Input: part model. Units: mm. Frame: model coordinates. A direction names the side the tool comes from. Coordinates: 2 decimals unless noted, no trailing zeros. Order: outer loops, then holes, each group sorted by start corner. A loop starts at its lowest first (then second) coordinate and runs counter-clockwise, first axis right, second up. Notation, with made-up numbers: M 48,-20 L 53,-20 A12 cw 53,-5 Z; hole C -8,35.5 d2. An arc over 180 degrees is marked long. One line per item, written item: value.
```python
from build123d import *

# Parameters (mm, degrees)
F0_W     = 18.0536359549
F0_H     = 24.487555027
F1_DEPTH = 48.0590760708
F2_R     = 4.7851705696
F3_DEPTH = 59.6192404628
F4_SIZE  = 5.08
F5_T     = -2.54


with BuildPart() as f1:
    # F0 (on Top) → F1 (new body)
    with BuildSketch(Plane.XY):
        with Locations((-3.9722770452, 28.8042277098)):
            Rectangle(F0_W, F0_H)
    extrude(amount=F1_DEPTH)

    # F2 (on face) → F3 (cut)
    with BuildSketch(Plane.YZ.offset(5.0545409322)):
        with Locations((27.5146439672, 27.5505185127)):
            Circle(F2_R)
    extrude(amount=-F3_DEPTH, mode=Mode.SUBTRACT)

    # F4
    f4_edges = [f1.edges().sort_by_distance(p)[0] for p in [
        (5.054541, 28.804228, 48.059076),
    ]]
    chamfer(f4_edges, length=F4_SIZE)

    # F5
    f5_openings = [f1.faces().sort_by_distance(p)[0] for p in [
        (-12.999095, 40.508625, 24.029538),
    ]]
    offset(amount=F5_T, openings=f5_openings)


solid = f1.part
```
(1) Draft query along Y for faces 1 (the flat face through (2.515, 29, 18)), 2 (the flat face through (-4, 41.048, 24)), 3 (the flat face through (-12.999, 29, 32.3)), 4 (the flat face through (-4, 16.56, 24)). Return one class per face: released by +Y, released by -Y, zero draft, split by the parting line, or undercut.
Data:
face 1: undercut
face 2: released by +Y
face 3: zero draft
face 4: released by -Y
(2) Ray query, line 1 (Y direction, x = 0.5, z = 39); line 2 (Z direction, x = -8.25, y = 37.75); line 3 (Z direction, x = 2.25, y = 31.25). Return the intervals inside material, ascending. Write a range as from..to.
Data:
line 1: y = 16.56..19.1, 38.51..41.05
line 2: z = 0..2.54, 45.52..48.06
line 3: z = 0..2.54, 21.25..24.56, 30.54..33.85, 42.19..45.78
(3) First-contact query: pin 1 (4 mm diameter, centred on y = 35, z = 20.5, fed in from -X). Flat tip, straight axial feed; report the tip coordinate or a pass-through.
Data:
pin 1: stops at x = 2.51
(4) Cut plane A-A on x = 0.75. Output: boundary loops of the cut face in (y, z).
Data:
outline: M 16.56,0 L 41.05,0 L 41.05,47.28 L 16.56,47.28 Z; C 27.51,27.55 d14.65; hole M 19.1,2.54 L 38.51,2.54 L 38.51,43.69 L 19.1,43.69 Z; hole C 27.51,27.55 d9.57
(5) Access query for faces 5 (the flat face through (-5, 38.508, 24)), 6 (the flat face through (2.55, 28.633, 45.484)). Directions: +Z, -Z, +X, -X, +Y, -Y. A direction counts if a zero-diameter tool reaches every point of the face in a straight line with its end or side. Return the directions, or none.
Data:
face 5: -X
face 6: +Z, +X, +Y, -Y
(6) Cut plane C-C on z = 15.5. Output: boundary loops of the cut face in (x, y).
Data:
outline: M -13,16.56 L 5.05,16.56 L 5.05,41.05 L -13,41.05 L -13,38.51 L 2.51,38.51 L 2.51,19.1 L -13,19.1 Z
(7) Cut plane D-D on x = -10.25. Output: boundary loops of the cut face in (y, z), plus the area to 3 significant figures.
Data:
outline: M 16.56,0 L 41.05,0 L 41.05,48.06 L 16.56,48.06 Z; C 27.51,27.55 d14.65; hole M 19.1,2.54 L 38.51,2.54 L 38.51,45.52 L 19.1,45.52 Z; hole C 27.51,27.55 d9.57
area: 439 mm2
(8) Cut plane B-B on y = 37. Output: boundary loops of the cut face in (x, z), plus the area to 3 significant figures.
Data:
outline: M -13,0 L 5.05,0 L 5.05,42.98 L -0.03,48.06 L -13,48.06 L -13,45.52 L -1.08,45.52 L 2.51,41.93 L 2.51,2.54 L -13,2.54 Z
area: 194 mm2
